For this review, take the finished solid that the model builds, in its own axes (mm). A direction names the side the tool comes from. Coordinates: 2 decimals unless noted, no trailing zeros. Loops run counter-clockwise (first coordinate to the right, second up) from the corner with the lowest first, then second, coordinate; pieces in that order, holes last. Notation, with made-up numbers: M 24.25,36 L 50.25,36 A33 ccw 50.25,74 Z; hole C -8.5,-26.75 d8. An arc over 180 degrees is marked long. Answer as a JSON object with one key per item and string values. Group by question number.
Item 1: Add section C-C (y = 17). State the section outline as (x, z) points, then the cut area to 3 significant figures.
Item 2: Mouldability with a two-part tool opening along Z and no side actions: class faces 1 (the face through (0, 15, 0)), 2 (the face through (-23, 0, 15)), 3 (the face through (23.5, 8, 15)), 4 (the face through (0, 15, 30)) as +Z half, -Z half, draft (parallel to the pull), parting line (faces both ways), or undercut.
Item 3: Add section D-D (z = 8). State the section outline as (x, y) points, then the cut area to 3 significant figures.
Item 4: Add section B-B (z = 15). State the section outline as (x, y) points, then the cut area to 3 significant figures.
Item 5: Insertion check: pin 1 (5 mm diameter, centred on x = 19.25, z = 15, fed in from -Y); pin 2 (4 mm diameter, centred on x = 8, z = 19, fed in from -Y); pin 3 (10.5 mm diameter, centred on x = 0, z = 15, fed in from -Y); pin 4 (2.5 mm diameter, centred on x = 18.5, z = 13, fed in from +Y). Each pin has a flat end and moves straight along its axis. Give the tip position at first contact, or say it passes through.
Item 6: Wall thickness on L1, parallel to Z at x = -19.25, y = 14; L2, parallel to Z at x = 0, y = 14.25; L3, parallel to X at y = 5.25, z = 19: over which ranges is each line inside the solid? List them lowest first. Write a range as from..to.
Item 7: Add section A-A (x = -1). State the section outline as (y, z) points, then the cut area to 3 significant figures.
Item 8: Tool access review of faces 5 (the face through (-22, 2, 15)), 6 (the face through (-3.802, 16.323, 21.465)), 7 (the face through (20.87, 9.38, 18.97)): name each direction out of +Z, -Z, +X, -X, +Y, -Y from which nothing blocks a thin tool from reaching the whole face with its end or side.
from build123d import *

# Parameters (mm, degrees)
PAD_DEPTH       = 30
SKETCH001_R     = 4
POCKET_DEPTH    = 26.001
POCKET001_DEPTH = 19.001
SKETCH003_R     = 2.75
POCKET002_DEPTH = 25.001
SKETCH004_R     = 4.75
POCKET003_DEPTH = 20.001


with BuildPart() as part:
    # Sketch → Pad (new body)
    with BuildSketch(Plane.XY):
        with BuildLine():
            Line((-25.980762, 0), (-14.96663, 0))
            ThreePointArc((14.96663, 0), (0, 14), (-14.96663, 0))
            Line((14.96663, 0), (25.980762, 0))
            ThreePointArc((25.980762, 0), (0, 25), (-25.980762, 0))
        make_face()
    extrude(amount=PAD_DEPTH)

    # Sketch001 (on DatumPlane) → Pocket (cut, through all)
    with BuildSketch(Plane(origin=(0, 26, 0), x_dir=(-1, 0, 0), z_dir=(0, 1, 0))):
        with Locations((0, 15)):
            Circle(SKETCH001_R)
    extrude(amount=-POCKET_DEPTH, mode=Mode.SUBTRACT)

    # Sketch002 (on DatumPlane) → Pocket001 (cut, through all)
    with BuildSketch(Plane(origin=(0, 19, 0), x_dir=(-1, 0, 0), z_dir=(0, 1, 0))):
        Polygon((0, 23.660254), (-7.5, 19.330127), (-7.5, 10.669873), (0, 6.339746), (7.5, 10.669873), (7.5, 19.330127), align=None)
    extrude(amount=-POCKET001_DEPTH, mode=Mode.SUBTRACT)

    # Sketch003 (on DatumPlane) → Pocket002 (cut, through all)
    with BuildSketch(Plane.XZ):
        with Locations((19.25, 15)):
            Circle(SKETCH003_R)
        with Locations((-19.25, 15)):
            Circle(SKETCH003_R)
    extrude(amount=-POCKET002_DEPTH, mode=Mode.SUBTRACT)

    # Sketch004 (on DatumPlane) → Pocket003 (cut, through all)
    with BuildSketch(Plane(origin=(0, 5, 0), x_dir=(-1, 0, 0), z_dir=(0, 1, 0))):
        with Locations((19.25, 15)):
            Circle(SKETCH004_R)
        Polygon((-19.25, 19.907477), (-23.5, 17.453739), (-23.5, 12.546261), (-19.25, 10.092523), (-15, 12.546261), (-15, 17.453739), align=None)
    extrude(amount=POCKET003_DEPTH, mode=Mode.SUBTRACT)


solid = part.part
From the geometry:
{
 "1": {"outline": "M -18.76,0 L 18.76,0 L 18.76,10.37 L 15,12.55 L 15,17.45 L 18.76,19.63 L 18.76,30 L -18.76,30 L -18.76,19.72 A4.75 cw -18.76,10.28 Z; hole M -7.5,10.67 L 0,6.34 L 7.5,10.67 L 7.5,19.33 L 0,23.66 L -7.5,19.33 Z", "area": "873 mm²"},
 "2": {"face 1": "-Z half", "face 2": "draft", "face 3": "undercut", "face 4": "+Z half"},
 "3": {"outline": "M -25.98,0 L -14.97,0 A15 cw -2.88,13.72 L -2.88,19 L 2.88,19 L 2.88,13.72 A15 cw 14.97,0 L 25.98,0 A26 ccw Z", "area": "657 mm²"},
 "4": {"outline": "M -25.98,0 L -22,0 L -22,5 L -24,5 L -24,9 A26 ccw Z; M -16.5,0 L -14.97,0 A15 cw -7.5,11.99 L -7.5,19 L -4,19 L -4,24.69 A26 ccw -14.5,20.58 L -14.5,5 L -16.5,5 Z; M 4,19 L 7.5,19 L 7.5,11.99 A15 cw 14.97,0 L 16.5,0 L 16.5,5 L 15,5 L 15,20.24 A26 ccw 4,24.69 Z; M 22,0 L 25.98,0 A26 ccw 23.5,10.12 L 23.5,5 L 22,5 Z", "area": "301 mm²"},
 "5": {"pin 1": "passes through", "pin 2": "stops at y = 10.18", "pin 3": "stops at y = 19", "pin 4": "stops at y = 5"},
 "6": {"L1": "z = 0..10.25, 19.75..30", "L2": "z = 0..6.34, 23.66..30", "L3": "x = -25.24..-21.81, -16.69..-13.64, 13.64..17.68, 20.82..25.24"},
 "7": {"outline": "M 13.97,0 L 24.98,0 L 24.98,11.13 L 19,11.13 L 19,6.92 L 13.97,6.92 Z; M 13.97,23.08 L 19,23.08 L 19,18.87 L 24.98,18.87 L 24.98,30 L 13.97,30 Z", "area": "203 mm²"},
 "8": {"face 5": "+Y, -Y", "face 6": "-Y", "face 7": "+Y"}
}
